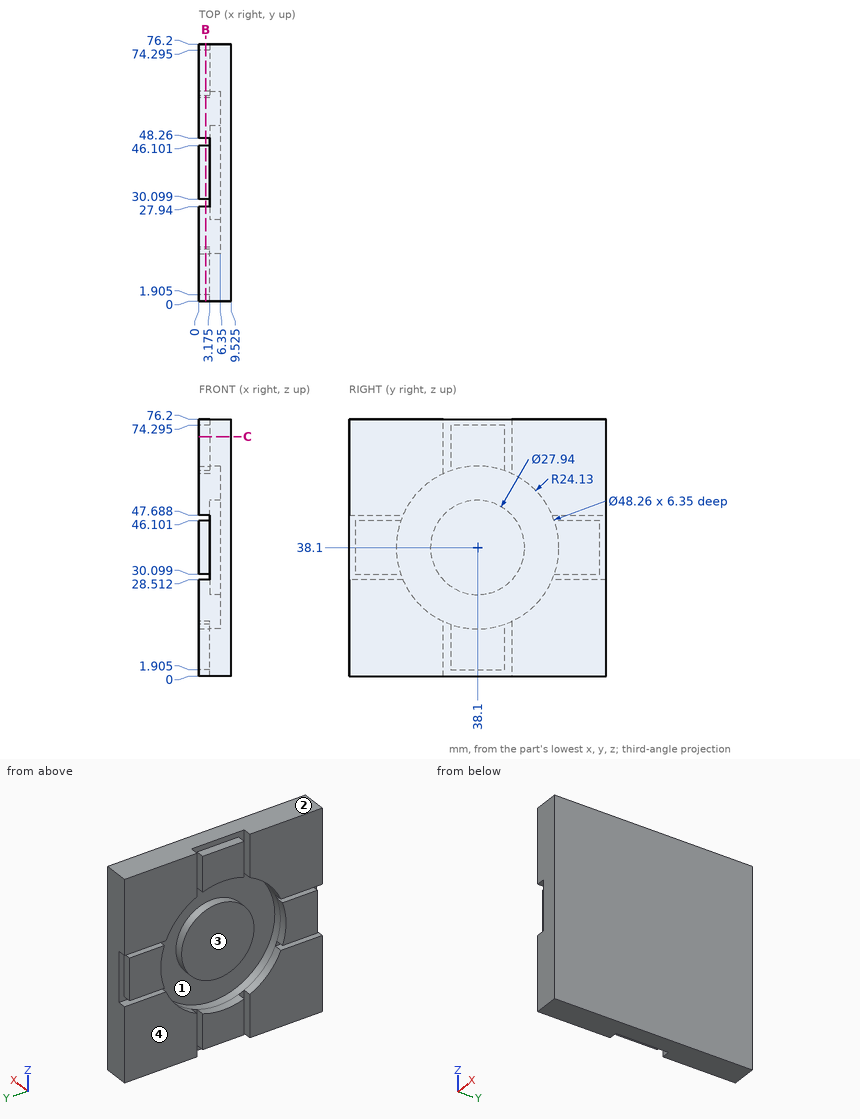
Source: three-view drawing plus pictorial views. Frame: mm from the lowest corner of the part. Give positions to 0.01 mm unless a question says otherwise; leave off trailing zeros. Order: outer loops, then holes, each group sorted by start corner. A loop starts at its lowest first (then second) coordinate and runs counter-clockwise, first axis right, second up.
1. Section C-C on z = 71. Return the cut outline in (x, y) (1 decimal), and give its area (3 significant figures).
Derived:
outline: (0, 0) - (9.5, 0) - (9.5, 76.2) - (0, 76.2) - (0, 48.3) - (3.2, 48.3) - (3.2, 46.1) - (0, 46.1) - (0, 30.1) - (3.2, 30.1) - (3.2, 27.9) - (0, 27.9) - close
area: 712 mm2
2. Pin query (flat end, axial travel): pin 1 (1.6 mm diameter, centred on x = 1, z = 40.5, fed in from +Y) (3 decimals); pin 2 (2.5 mm diameter, centred on x = 1.5, y = 40.5, fed in from -Z) (3 decimals). Return the tip coordinate at first contact, or that it passes through.
Derived:
pin 1: stops at y = 74.295
pin 2: stops at z = 1.905
3. Material intervals for L1, parallel to Y at x = 3.25, z = 28.5; L2, parallel to Y at x = 2.5, z = 8.5; L3, parallel to Z at x = 1.75, y = 67, sorted ascending.
Derived:
L1: y = 0 to 15.96, 27.95 to 48.25, 60.24 to 76.2
L2: y = 0 to 27.94, 30.1 to 46.1, 48.26 to 76.2
L3: z = 0 to 28.51, 30.1 to 46.1, 47.69 to 76.2
4. Mould query, pull axis Z, two halves, no side actions, for the marked faces 1, 2, 3 and 4. Classes: released by +Z, released by -Z, zero draft, split by the parting line, or undercut.
Derived:
face 1: undercut
face 2: released by +Z
face 3: undercut
face 4: zero draft
5. Section B-B on x = 2. Give the number of separate pieces and of enclosed holes in the cut face, and give its area (3 significant figures).
Derived:
separate pieces: 8
enclosed holes: 0
area: 3,620 mm2
